Source: CAD feature listing. Evaluate the final solid. Frame: model axes, mm. Round coordinates to 2 decimals unless told otherwise and drop trailing zeros. Order: outer loops, then holes, each group sorted by start corner. A loop starts at its lowest first (then second) coordinate and runs counter-clockwise, first axis right, second up.
```python
from build123d import *

# Parameters (mm, degrees)
F0_R     = 0.9017
F0_R_2   = 2.286
F1_DEPTH = 3.6322


with BuildPart() as f1:
    # F0 (on Top) → F1 (new body)
    with BuildSketch(Plane.XY):
        with BuildLine():
            Line((25.000407, 6.947678), (1.864265, 10.903473))
            ThreePointArc((1.864265, 10.903473), (0, 11.0617), (-1.864265, 10.903473))
            Line((-1.864265, 10.903473), (-25.000407, 6.947678))
            ThreePointArc((-25.000407, 6.947678), (-30.861, 0), (-25.000407, -6.947678))
            Line((-25.000407, -6.947678), (-1.864265, -10.903473))
            ThreePointArc((-1.864265, -10.903473), (0, -11.0617), (1.864265, -10.903473))
            Line((1.864265, -10.903473), (25.000407, -6.947678))
            ThreePointArc((25.000407, -6.947678), (30.861, 0), (25.000407, 6.947678))
        make_face()
        with Locations((5.352233, -5.352233)):
            Circle(F0_R, mode=Mode.SUBTRACT)
        with Locations((-23.8125, 0)):
            Circle(F0_R_2, mode=Mode.SUBTRACT)
        with BuildLine():
            ThreePointArc((-4.450533, 5.352233), (-4.51917, 5.007167), (-4.714634, 4.714634))
            ThreePointArc((-4.714634, 4.714634), (-6.185295, 5.697298), (-4.450533, 5.352233))
        make_face(mode=Mode.SUBTRACT)
        with BuildLine():
            ThreePointArc((-2.298946, 2.298946), (1.24418, 3.003717), (3.2512, 0))
            ThreePointArc((3.2512, 0), (-1.24418, -3.003717), (-2.298946, 2.298946))
        make_face(mode=Mode.SUBTRACT)
        with Locations((23.8125, 0)):
            Circle(F0_R_2, mode=Mode.SUBTRACT)
    extrude(amount=F1_DEPTH)


solid = f1.part
```
1. First-contact query: pin 1 (4 mm diameter, centred on x = -23.81, y = 0, fed in from +Z); pin 2 (1 mm diameter, centred on x = 6, z = 3, fed in from +Y). Flat tips, straight axial feed; report the tip coordinate or a pass-through.
2. Section B-B on x = 0. Return loops of the section in (y, z), plus the area to 3 significant figures.
3. Section A-A on y = 1. Return loops of the section in (x, z).
4. Section D-D on x = 7. Return loops of the section in (y, z).
5. Pull-direction query (X, two-part tool) for faces 1 (the face through (-13, 9, 2)), 2 (the face through (-21.701, -0.876, 1.791)), 3 (the face through (13.59, 8.9, 1.79)); classes: released by +X, released by -X, zero draft, split by the parting line, or undercut.
6. Line query: line 1 along X through (y, z) = (-1.25, 1.15); line 2 along X through (y, z) = (0.75, 2.2); line 3 along Y through (x, z) = (-1, 3). Output: solid intervals per line, ascending.
7. Section C-C on z = 2.95. Return loops of the section in (x, y), plus the area to 3 significant figures.
Result:
1. pin 1: passes through
1. pin 2: stops at y = 10.28
2. outline: (-11.06, 0) - (-3.25, 0) - (-3.25, 3.63) - (-11.06, 3.63) - close; (3.25, 0) - (11.06, 0) - (11.06, 3.63) - (3.25, 3.63) - close
2. area: 56.7 mm2
3. outline: (-30.79, 0) - (-25.87, 0) - (-25.87, 3.63) - (-30.79, 3.63) - close; (-21.76, 0) - (-3.09, 0) - (-3.09, 3.63) - (-21.76, 3.63) - close; (3.09, 0) - (21.76, 0) - (21.76, 3.63) - (3.09, 3.63) - close; (25.87, 0) - (30.79, 0) - (30.79, 3.63) - (25.87, 3.63) - close
4. outline: (-10.03, 0) - (10.03, 0) - (10.03, 3.63) - (-10.03, 3.63) - close
5. face 1: released by -X
5. face 2: undercut
5. face 3: released by +X
6. line 1: x = -30.75 to -25.73, -21.9 to -3, 3 to 21.9, 25.73 to 30.75
6. line 2: x = -30.82 to -25.97, -21.65 to -3.16, 3.16 to 21.65, 25.97 to 30.82
6. line 3: y = -11.02 to -3.09, 3.09 to 11.02
7. outline: (-25, -6.95) - (-1.86, -10.9) arc R11.06 ccw to (1.86, -10.9) - (25, -6.95) arc R7.05 ccw to (25, 6.95) - (1.86, 10.9) arc R11.06 ccw to (-1.86, 10.9) - (-25, 6.95) arc R7.05 ccw to start; hole circle Ø4.57 at (-23.81, 0); hole (-4.71, 4.71) arc R0.9 ccw to (-4.45, 5.35) arc R0.9 ccw (long way) to start; hole (-2.3, 2.3) arc R3.25 ccw (long way) to (3.25, 0) arc R3.25 ccw to start; hole circle Ø1.8 at (5.35, -5.35); hole circle Ø4.57 at (23.81, 0)
7. area: 960 mm2
